Could you check a few things on this model? Use its own coordinates, in mm. A direction names the side the tool comes from. Round coordinates to 2 decimals unless told otherwise and drop trailing zeros. Order: outer loops, then holes, each group sorted by start corner. A loop starts at its lowest first (then second) coordinate and runs counter-clockwise, first axis right, second up. Notation, with made-up numbers: M -11,79 L 21,79 A5 cw 21,86 Z; hole C 36.5,1.25 d4. An arc over 180 degrees is marked long. Write each question's results on one line, items separated by ' | '. Start each with the question number.
1. I'm going to push flat-ended pins straight in: pin 1 (7.5 mm diameter, centred on x = -14, y = 46.5, fed in from +Z); pin 2 (3 mm diameter, centred on x = -13.5, y = 66.5, fed in from +Z); pin 3 (2 mm diameter, centred on x = -71, y = 38.5, fed in from +Z). Where does each tip first touch, or does it pass through?
2. Suppose I cut it at A-A on z = 9. Write out the boundary of the cut face in (x, y), and give its area (3 significant figures).
3. Suppose I cut it at C-C on z = 82.5. Write out the boundary of the cut face in (x, y), and give its area (3 significant figures).
4. Suppose I cut it at D-D on x = -110.5. Write out the boundary of the cut face in (y, z), and give its area (3 significant figures).
5. Please list where these lines run through material, in increasing order: L1, parallel to Y at x = -82.5, z = 64; L2, parallel to Y at x = -112, z = 49; L3, parallel to Y at x = -45, z = 6.
6. Suppose I cut it at B-B on z = 58. Write out the boundary of the cut face in (x, y), and give its area (3 significant figures).
7. We'd pull the mould along Y, two halves only. Please class faces 1 (the flat face through (-36, 64.887, 45)), 2 (the flat face through (-135.848, 39, 23)), 3 (the flat face through (-36, 123.444, 56)): released by +Y, released by -Y, zero draft, split by the parting line, or undercut.
8. For faces 4 (the flat face through (-36, 101.895, 58)), 5 (the flat face through (-36, 63, 0)), which set-ups out of +Z, -Z, +X, -X, +Y, -Y let a thin tool reach every point of the face, with its end or its side?
from build123d import *

# Parameters (mm, degrees)
SKETCH_W     = 203.2
SKETCH_H     = 203.2
PAD_DEPTH    = 2.54
SKETCH001_W  = 203.2
SKETCH001_H  = 2.54
PAD001_DEPTH = 111.506
SKETCH002_W  = 203.2
SKETCH002_H  = 2.54
PAD002_DEPTH = 86.106
SKETCH003_W  = 203.2
SKETCH003_H  = 2.54
PAD003_DEPTH = 60.706
SKETCH004_W  = 203.2
SKETCH004_H  = 2.54
PAD004_DEPTH = 35.306
SKETCH007_W  = 227.037744
SKETCH007_H  = 43.51487
POCKET_DEPTH = 80.01


with BuildPart() as part:
    # Sketch (on XY_Plane of Origin) → Pad (new body)
    with BuildSketch(Plane.XY):
        with Locations((-34.247654, 21.844)):
            Rectangle(SKETCH_W, SKETCH_H)
    extrude(amount=PAD_DEPTH)

    # Sketch001 (on Face6 of Pad) → Pad001 (join)
    with BuildSketch(Plane.XY.offset(2.54)):
        with Locations((-34.247654, 122.174)):
            Rectangle(SKETCH001_W, SKETCH001_H)
        with Locations((-34.247654, 100.624772)):
            Rectangle(SKETCH001_W, SKETCH001_H)
    extrude(amount=PAD001_DEPTH)

    # Sketch002 (on Face6 of Pad001) → Pad002 (join)
    with BuildSketch(Plane.XY.offset(2.54)):
        with Locations((-34.247654, 66.156921)):
            Rectangle(SKETCH002_W, SKETCH002_H)
    extrude(amount=PAD002_DEPTH)

    # Sketch003 (on Face11 of Pad002) → Pad003 (join)
    with BuildSketch(Plane.XY.offset(2.54)):
        with Locations((-34.247654, 38.216921)):
            Rectangle(SKETCH003_W, SKETCH003_H)
    extrude(amount=PAD003_DEPTH)

    # Sketch004 (on Face15 of Pad003) → Pad004 (join)
    with BuildSketch(Plane.XY.offset(2.54)):
        with Locations((-34.247654, 1.27)):
            Rectangle(SKETCH004_W, SKETCH004_H)
    extrude(amount=PAD004_DEPTH)

    # Sketch007 → Pocket (cut)
    with BuildSketch(Plane.XZ.offset(79.756)):
        with Locations((-24.815948, 21.757435)):
            Rectangle(SKETCH007_W, SKETCH007_H)
    extrude(amount=-POCKET_DEPTH, mode=Mode.SUBTRACT)


solid = part.part
Filled sheet:
1) pin 1: stops at z = 2.54 | pin 2: stops at z = 88.65 | pin 3: stops at z = 63.25
2) outline: M -135.85,0.25 L 67.35,0.25 L 67.35,2.54 L -135.85,2.54 Z; M -135.85,36.95 L 67.35,36.95 L 67.35,39.49 L -135.85,39.49 Z; M -135.85,64.89 L 67.35,64.89 L 67.35,67.43 L -135.85,67.43 Z; M -135.85,99.35 L 67.35,99.35 L 67.35,101.89 L -135.85,101.89 Z; M -135.85,120.9 L 67.35,120.9 L 67.35,123.44 L -135.85,123.44 Z | area: 2,530 mm^2
3) outline: M -135.85,64.89 L 67.35,64.89 L 67.35,67.43 L -135.85,67.43 Z; M -135.85,99.35 L 67.35,99.35 L 67.35,101.89 L -135.85,101.89 Z; M -135.85,120.9 L 67.35,120.9 L 67.35,123.44 L -135.85,123.44 Z | area: 1,550 mm^2
4) outline: M 0.25,0 L 123.44,0 L 123.44,114.05 L 120.9,114.05 L 120.9,2.54 L 101.89,2.54 L 101.89,114.05 L 99.35,114.05 L 99.35,2.54 L 67.43,2.54 L 67.43,88.65 L 64.89,88.65 L 64.89,2.54 L 39.49,2.54 L 39.49,63.25 L 36.95,63.25 L 36.95,2.54 L 2.54,2.54 L 2.54,37.85 L 0.25,37.85 Z | area: 1,330 mm^2
5) L1: y = 64.89 to 67.43, 99.35 to 101.89, 120.9 to 123.44 | L2: y = 36.95 to 39.49, 64.89 to 67.43, 99.35 to 101.89, 120.9 to 123.44 | L3: y = 0.25 to 2.54, 36.95 to 39.49, 64.89 to 67.43, 99.35 to 101.89, 120.9 to 123.44
6) outline: M -135.85,36.95 L 67.35,36.95 L 67.35,39.49 L -135.85,39.49 Z; M -135.85,64.89 L 67.35,64.89 L 67.35,67.43 L -135.85,67.43 Z; M -135.85,99.35 L 67.35,99.35 L 67.35,101.89 L -135.85,101.89 Z; M -135.85,120.9 L 67.35,120.9 L 67.35,123.44 L -135.85,123.44 Z | area: 2,060 mm^2
7) face 1: undercut | face 2: zero draft | face 3: released by +Y
8) face 4: +Z, +X, -X | face 5: -Z, +X, -X, +Y, -Y
